Could you check a few things on this model? Use its own coordinates, in mm. A direction names the side the tool comes from. Coordinates: 2 decimals unless noted, no trailing zeros. Order: outer loops, then holes, each group sorted by start corner. A loop starts at its lowest first (then second) coordinate and runs counter-clockwise, first axis right, second up. Notation, with made-up numbers: (86.5, 10.5) - (116.5, 10.5) arc R11 ccw to (116.5, 15.5) - close; hole circle Ø10 at (-36.75, 26.5). An arc over 180 degrees is marked (long way). Answer as a JSON object with one key per item and string values. Group by question number.
(1) Please list where these lines run through material, in increasing order: probe 1 along Z at (x, y) = (-142.5, 48); probe 2 along X at (y, z) = (51.5, 20); probe 3 along X at (y, z) = (3.5, 171).
(2) We'd pull the mould along X, two halves only. Please class faces 1 (the cylindrical face through (-95.96, 15.37, 196.38)), 2 (the cylindrical face through (-194.21, 3.06, 93.67)), 3 (the flat face through (-100, 0, 94)): pulls with the +X half, pulls with the -X half, needs draft (parallel to the pull), parting line crosses it, or undercut.
(3) Imagine slicing it at A-A, the plane y = 33. Write out the boundary of the cut face in (x, z), and give its area (3 significant figures).
(4) Imagine slicing it at D-D, the plane x = -145.5. Write out the boundary of the cut face in (y, z).
(5) Imagine slicing it at C-C, the plane y = 13. Write out the boundary of the cut face in (x, z).
(6) Which directions (+Z, -Z, +X, -X, +Y, -Y) give clear straight access to the entire face, cutting with the end or side of a thin tool? Please do faces 4 (the cylindrical face through (-165.3, 38.2, 196.4)), 5 (the flat face through (-160, 28, 202.946)).
(7) Will this pin go through, and if not, where does the flat tip stop? P1, Ø6, axis at x = -78, y = 36, coming from the +Z side.
(8) Imagine slicing it at B-B, the plane x = -105. Write out the boundary of the cut face in (y, z), and give its area (3 significant figures).
from build123d import *

# Parameters (mm, degrees)
SKETCH1_W           = 197.104
SKETCH1_H           = 189.992
BOSS_EXTRUDE1_DEPTH = 59.944
FILLET1_R           = 10.16
FILLET2_R           = 10.16
FILLET3_R           = 10.16
FILLET4_R           = 10.16
SKETCH2_R           = 10.892824913
SKETCH2_R_2         = 6.956698316
SKETCH2_R_3         = 6.871617304
BOSS_EXTRUDE3_DEPTH = 12.954


with BuildPart() as part:
    # Sketch1 → Boss-Extrude1 (new body)
    with BuildSketch(Plane(origin=(0, 0, 0), x_dir=(1, 0, 0), z_dir=(0, 1, 0))):
        with Locations((-98.552, -94.996)):
            Rectangle(SKETCH1_W, SKETCH1_H)
    extrude(amount=BOSS_EXTRUDE1_DEPTH)

    # Fillet1
    fillet1_edges = [part.edges().sort_by_distance(p)[0] for p in [
        (0, 59.944, 94.996),
    ]]
    fillet(fillet1_edges, radius=FILLET1_R)

    # Fillet2
    fillet2_edges = [part.edges().sort_by_distance(p)[0] for p in [
        (0, 0, 94.996),
    ]]
    fillet(fillet2_edges, radius=FILLET2_R)

    # Fillet3
    fillet3_edges = [part.edges().sort_by_distance(p)[0] for p in [
        (-197.104, 59.944, 94.996),
    ]]
    fillet(fillet3_edges, radius=FILLET3_R)

    # Fillet4
    fillet4_edges = [part.edges().sort_by_distance(p)[0] for p in [
        (-197.104, 0, 94.996),
    ]]
    fillet(fillet4_edges, radius=FILLET4_R)

    # Sketch2 → Boss-Extrude3 (add)
    with BuildSketch(Plane.XY.offset(189.992)):
        with Locations(Location((-160.289066684, 28.528637542, 0), (0, 0, 180))):
            Circle(SKETCH2_R)
        with Locations(Location((-102.910266874, 15.674726269, 0), (0, 0, 180))):
            Circle(SKETCH2_R_2)
        with Locations(Location((-38.243166858, 15.674726269, 0), (0, 0, 180))):
            Circle(SKETCH2_R_3)
    extrude(amount=BOSS_EXTRUDE3_DEPTH)


solid = part.part
Result set:
{
 "1": {"probe 1": "z = 0 to 189.99", "probe 2": "x = -196.96 to -0.15", "probe 3": "x = -194.62 to -2.49"},
 "2": {"face 1": "undercut", "face 2": "pulls with the -X half", "face 3": "needs draft"},
 "3": {"outline": "(-197.1, 0) - (0, 0) - (0, 189.99) - (-150.36, 189.99) - (-150.36, 202.95) - (-170.22, 202.95) - (-170.22, 189.99) - (-197.1, 189.99) - close", "area": "37,700 mm^2"},
 "4": {"outline": "(0, 0) - (59.94, 0) - (59.94, 189.99) - (0, 189.99) - close"},
 "5": {"outline": "(-197.1, 0) - (0, 0) - (0, 189.99) - (-31.91, 189.99) - (-31.91, 202.95) - (-44.57, 202.95) - (-44.57, 189.99) - (-96.49, 189.99) - (-96.49, 202.95) - (-109.33, 202.95) - (-109.33, 189.99) - (-197.1, 189.99) - close"},
 "6": {"face 4": "+Z", "face 5": "+Z, +X, -X, +Y, -Y"},
 "7": {"P1": "stops at z = 189.99"},
 "8": {"outline": "(0, 0) - (59.94, 0) - (59.94, 189.99) - (22.31, 189.99) - (22.31, 202.95) - (9.04, 202.95) - (9.04, 189.99) - (0, 189.99) - close", "area": "11,600 mm^2"}
}
